Source: three-view drawing plus pictorial views. Frame: mm from the lowest corner of the part. A direction names the side the tool comes from. Coordinates: 2 decimals unless noted, no trailing zeros. Loops run counter-clockwise (first coordinate to the right, second up) from the corner with the lowest first, then second, coordinate; pieces in that order, holes last.
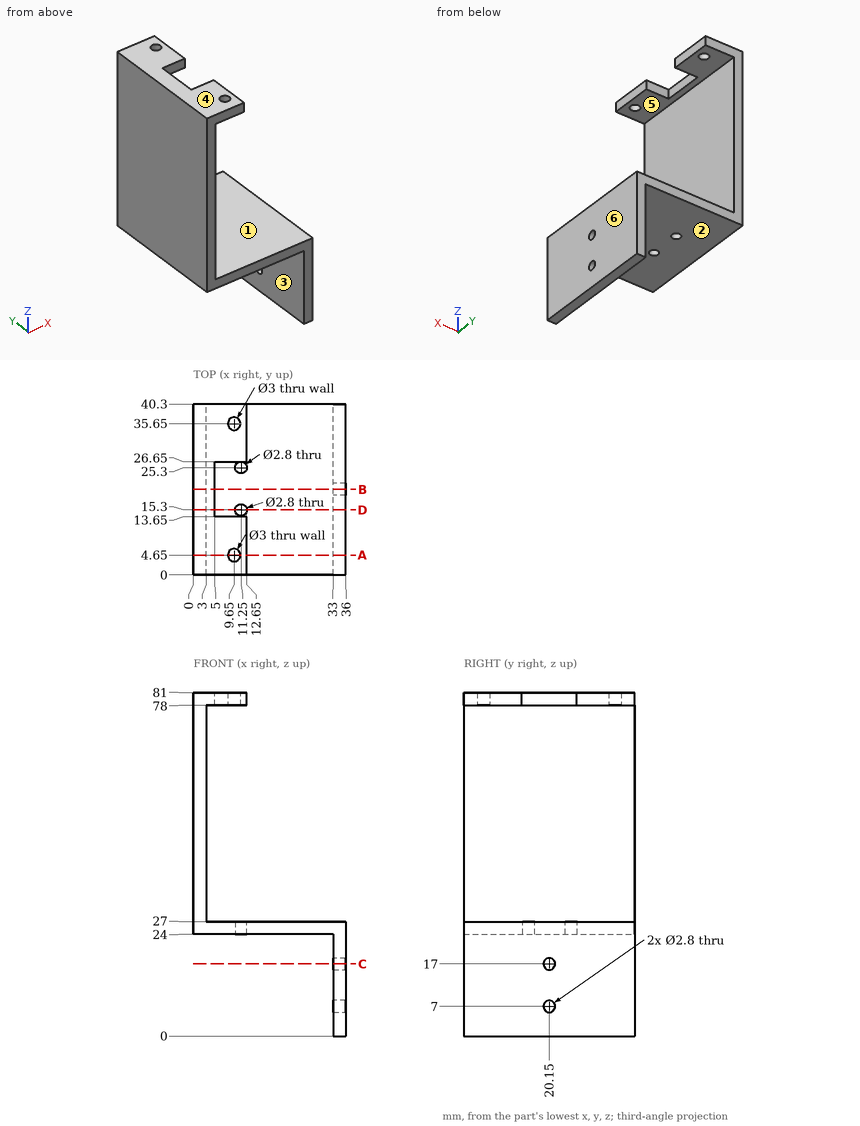
Q1. Section query B-B on y = 20.15. Return the cut outline in (x, z).
Q2. First-contact query: pin 1 Ø10 at (x, z) = (9.5, 54.5) entering from -Y; pin 2 Ø2.5 at (y, z) = (31.5, 79.5) entering from +X; pin 3 Ø3.5 at (x, y) = (9.65, 35.65) entering from -Z; pin 4 Ø1 at (x, y) = (23.5, 27.5) entering from +Z. Flat tips, straight axial feed; report the tip coordinate or a pass-through.
Q3. Draft query along Z for the marked faces 1, 2, 3 and 4. Return one class per face: released by +Z, released by -Z, zero draft, split by the parting line, or undercut.
Q4. Reachability of the marked faces 5 and 6 from +Z, -Z, +X, -X, +Y, -Y: full face, straight path, thin tool, end or side. Return the list, or none.
Q5. Section query A-A on y = 4.65. Return the cut outline in (x, z).
Q6. Section query D-D on y = 15.3. Return the cut outline in (x, z).
Q7. Section query C-C on z = 17. Return the cut outline in (x, y).
Q8. Material intervals for line 1 along Y through (x, z) = (9.65, 80.25); line 2 along Y through (x, z) = (11.25, 25.8); line 3 along Y through (x, z) = (35, 7), sorted ascending.
Resolved:
1. outline: (0, 24) - (33, 24) - (33, 18.4) - (36, 18.4) - (36, 27) - (3, 27) - (3, 78) - (5, 78) - (5, 81) - (0, 81) - close; (33, 0) - (36, 0) - (36, 5.6) - (33, 5.6) - close; (33, 8.4) - (36, 8.4) - (36, 15.6) - (33, 15.6) - close
2. pin 1: passes through
2. pin 2: stops at x = 12.65
2. pin 3: stops at z = 24
2. pin 4: stops at z = 27
3. face 1: undercut
3. face 2: released by -Z
3. face 3: zero draft
3. face 4: released by +Z
4. face 5: +X, +Y, -Y
4. face 6: +Z, -Z, +X, +Y, -Y
5. outline: (0, 24) - (33, 24) - (33, 0) - (36, 0) - (36, 27) - (3, 27) - (3, 78) - (8.15, 78) - (8.15, 81) - (0, 81) - close; (11.15, 78) - (12.65, 78) - (12.65, 81) - (11.15, 81) - close
6. outline: (0, 24) - (9.85, 24) - (9.85, 27) - (3, 27) - (3, 78) - (5, 78) - (5, 81) - (0, 81) - close; (12.65, 24) - (33, 24) - (33, 0) - (36, 0) - (36, 27) - (12.65, 27) - close
7. outline: (33, 0) - (36, 0) - (36, 18.75) - (33, 18.75) - close; (33, 21.55) - (36, 21.55) - (36, 40.3) - (33, 40.3) - close
8. line 1: y = 0 to 3.15, 6.15 to 13.65, 26.65 to 34.15, 37.15 to 40.3
8. line 2: y = 0 to 13.9, 16.7 to 23.9, 26.7 to 40.3
8. line 3: y = 0 to 18.75, 21.55 to 40.3
